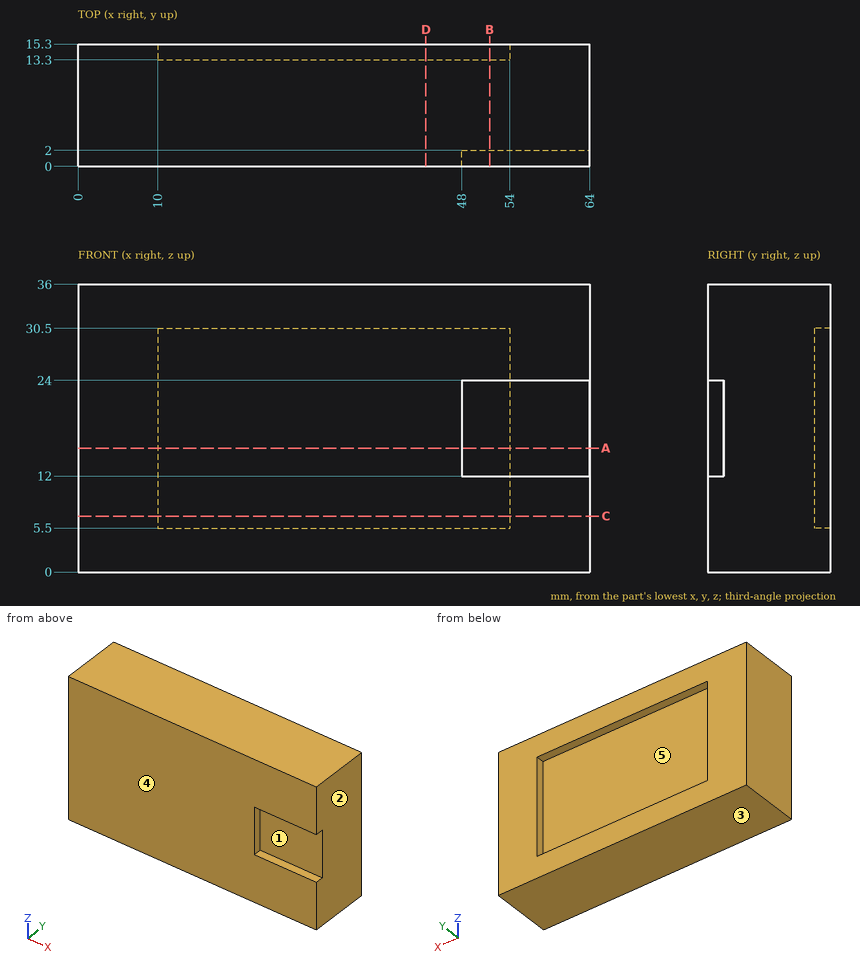
For this review, use the dimensioned drawing (mm, ordinates from the lowest corner) and the shaded views. A direction names the side the tool comes from. Coordinates: 2 decimals unless noted, no trailing zeros. Loops run counter-clockwise (first coordinate to the right, second up) from the corner with the lowest first, then second, coordinate; pieces in that order, holes last. Notation, with made-up numbers: (79.25, 33.25) -> (124.25, 33.25) arc R27 ccw to (124.25, 63.25) -> close; hole circle Ø1 at (-35.5, -17.75). An arc over 180 degrees is marked (long way). Return JSON: item names as keys, results as strings. Group by question number.
(1) For pin 1 Ø3.5 at (x, z) = (54.5, 20.5) entering from -Y; pin 2 Ø12.5 at (x, z) = (24.5, 19.5) entering from +Y; pin 3 Ø0.6 at (y, z) = (1, 20.5) entering from +X, all flat-tipped, find the tip position at first contact; note any pin that passes through.
(2) Consider section C-C, the plane z = 7. Give the boundary of the cut face in (x, y), plus the area to 3 significant figures.
(3) To check wall thickness, follow L1, parallel to X at y = 14.5, z = 13.5; L2, parallel to Z at x = 34, y = 14; L3, parallel to Y at x = 17, z = 26. State the ranges of each line that lie inside material, in increasing order.
(4) Tool access review of the marked faces 1 and 2: name each direction out of +Z, -Z, +X, -X, +Y, -Y from which nothing blocks a thin tool from reaching the whole face with its end or side.
(5) Consider section A-A, the plane z = 15.5. Give the boundary of the cut face in (x, y), plus the area to 3 significant figures.
(6) Mouldability with a two-part tool opening along Z and no side actions: class the marked faces 3, 4 and 5 as pulls with the +Z half, pulls with the -Z half, needs draft (parallel to the pull), parting line crosses it, or undercut.
(7) Consider section D-D, the plane x = 43.5. Give the boundary of the cut face in (y, z), plus the area to 3 significant figures.
(8) Consider section B-B, the plane x = 51.5. Give the boundary of the cut face in (y, z).
Results below:
{
 "1": {"pin 1": "stops at y = 2", "pin 2": "stops at y = 13.3", "pin 3": "stops at x = 48"},
 "2": {"outline": "(0, 0) -> (64, 0) -> (64, 15.3) -> (54, 15.3) -> (54, 13.3) -> (10, 13.3) -> (10, 15.3) -> (0, 15.3) -> close", "area": "891 mm2"},
 "3": {"L1": "x = 0 to 10, 54 to 64", "L2": "z = 0 to 5.5, 30.5 to 36", "L3": "y = 0 to 13.3"},
 "4": {"face 1": "+X, -Y", "face 2": "+Z, -Z, +X, +Y, -Y"},
 "5": {"outline": "(0, 0) -> (48, 0) -> (48, 2) -> (64, 2) -> (64, 15.3) -> (54, 15.3) -> (54, 13.3) -> (10, 13.3) -> (10, 15.3) -> (0, 15.3) -> close", "area": "859 mm2"},
 "6": {"face 3": "pulls with the -Z half", "face 4": "needs draft", "face 5": "undercut"},
 "7": {"outline": "(0, 0) -> (15.3, 0) -> (15.3, 5.5) -> (13.3, 5.5) -> (13.3, 30.5) -> (15.3, 30.5) -> (15.3, 36) -> (0, 36) -> close", "area": "501 mm2"},
 "8": {"outline": "(0, 0) -> (15.3, 0) -> (15.3, 5.5) -> (13.3, 5.5) -> (13.3, 30.5) -> (15.3, 30.5) -> (15.3, 36) -> (0, 36) -> (0, 24) -> (2, 24) -> (2, 12) -> (0, 12) -> close"}
}
